Autodesk Inventor part; units mm, degrees
ref_plane "YZ Plane" through (0, 0, 0) normal (1, 0, 0) x (0, 1, 0)
ref_plane "XZ Plane" through (0, 0, 0) normal (0, 1, 0) x (-1, 0, 0)
ref_plane "XY Plane" through (0, 0, 0) normal (0, 0, 1) x (1, 0, 0)
sketch "Sketch1" plane through (0, 0, 0) normal (0, 0, 1) x (1, 0, 0)
  line L0 (125, -40) -> (-125, -40)
  line L1 (-125, -40) -> (-125, 40)
  line L2 (-125, 40) -> (125, 40)
  line L3 (125, 40) -> (125, -40)
  line L4 (0, 56) -> (0, -56) construction
  line L5 (-175, 0) -> (175, 0) construction
  point P0 (0, 0)
  dimension "d0" = 250
  dimension "d1" = 80
extrude "Extrusion1" add sketch "Sketch1" along normal mid plane 3.175
sketch "Sketch2" plane through (0, 0, 1.5875) normal (0, 0, 1) x (1, 0, 0)
  line L0 (0, 56) -> (0, -56) construction
  line L1 (-175, 0) -> (175, 0) construction
  line L2 (-125, -40) -> (125, -40)
  circle A0 centre (-40, 0) radius 17.5
  circle A1 centre (40, 0) radius 17.5
  line L3 (-40, -28.575) -> (-40, 28.575) construction
  circle A2 centre (-40, 28.575) radius 4.5
  circle A3 centre (-40, -28.575) radius 4.5
  circle A4 centre (40, -28.575) radius 4.5
  circle A5 centre (40, 28.575) radius 4.5
  point P0 (0, 0)
  dimension "d4" = 40
  dimension "d5" = 80
  dimension "d6" = 35
  dimension "d7" = 57.15
  dimension "d8" = 9
extrude "Extrusion2" cut sketch "Sketch2" against normal up to surface (3.175 mm away)
chamfer "Chamfer1" distance 10 angle 45 2 edges at (125, 40, 0) (-125, 40, 0)
properties part number "Pedalbox_V2_Vert_Rectangle"
Design review of the part built by this model. Coordinates are the model's own, in mm. Coordinates: 2 decimals unless noted, no trailing zeros. Order: outer loops, then holes, each group sorted by start corner. A loop starts at its lowest first (then second) coordinate and runs counter-clockwise, first axis right, second up. Notation, with made-up numbers: (51, 70) -> (100, 70) arc R11 ccw to (100, 78) -> close; hole circle Ø4 at (5.25, 36.25). An arc over 180 degrees is marked (long way). Use one line per item in the form item = value. Start each with the question number.
(1) Add section B-B on x = -40. State the section outline as (y, z) points (1 decimal).
(2) Add section A-A on y = 0. State the section outline as (x, z) points.
(3) Add section D-D on x = 53. State the section outline as (y, z) points.
(4) The part is to be moulded in two halves that separate along X. For faces 1 (the flat face through (-2, 1, 1.588)), 2 (the cylindrical face through (44.3, 29.9, 0)), 3 (the flat face through (-120, 35, 0)), say which applies: +X half, -X half, draft (parallel to the pull), parting line (faces both ways), or undercut.
(5) Add section C-C on z = -1.1. State the section outline as (x, y) points (3 decimals).
(6) For probe 1 along Y at (x, z) = (40, -0.2) (3 decimals); probe 2 along Y at (x, z) = (-37, 1.05); probe 3 along X at (y, z) = (-6, 0.25), list the stretches that pass through material, from the lowest coordinate up.
(7) Insertion check: pin 1 (8 mm diameter, centred on x = 40, y = -28.575, fed in from +Z); pin 2 (14.5 mm diameter, centred on x = -40, y = -28.575, fed in from +Z). Each pin has a flat end and moves straight along its axis. Give the tip position at first contact, or say it passes through.
Answer block:
q1.outline = (-40, -1.6) -> (-33.1, -1.6) -> (-33.1, 1.6) -> (-40, 1.6) -> close; (-24.1, -1.6) -> (-17.5, -1.6) -> (-17.5, 1.6) -> (-24.1, 1.6) -> close; (17.5, -1.6) -> (24.1, -1.6) -> (24.1, 1.6) -> (17.5, 1.6) -> close; (33.1, -1.6) -> (40, -1.6) -> (40, 1.6) -> (33.1, 1.6) -> close
q2.outline = (-125, -1.59) -> (-57.5, -1.59) -> (-57.5, 1.59) -> (-125, 1.59) -> close; (-22.5, -1.59) -> (22.5, -1.59) -> (22.5, 1.59) -> (-22.5, 1.59) -> close; (57.5, -1.59) -> (125, -1.59) -> (125, 1.59) -> (57.5, 1.59) -> close
q3.outline = (-40, -1.59) -> (-11.72, -1.59) -> (-11.72, 1.59) -> (-40, 1.59) -> close; (11.72, -1.59) -> (40, -1.59) -> (40, 1.59) -> (11.72, 1.59) -> close
q4.face_1 = draft
q4.face_2 = undercut
q4.face_3 = -X half
q5.outline = (-125, -40) -> (125, -40) -> (125, 30) -> (115, 40) -> (-115, 40) -> (-125, 30) -> close; hole circle Ø35 at (-40, 0); hole circle Ø9 at (-40, -28.575); hole circle Ø9 at (-40, 28.575); hole circle Ø35 at (40, 0); hole circle Ø9 at (40, -28.575); hole circle Ø9 at (40, 28.575)
q6.probe_1 = -40 to -33.075, -24.075 to -17.5, 17.5 to 24.075, 33.075 to 40
q6.probe_2 = -40 to -31.93, -25.22 to -17.24, 17.24 to 25.22, 31.93 to 40
q6.probe_3 = -125 to -56.44, -23.56 to 23.56, 56.44 to 125
q7.pin_1 = through
q7.pin_2 = 1.59
